Autodesk Inventor part; units mm, degrees
ref_plane "YZ Plane" through (0, 0, 0) normal (1, 0, 0) x (0, 1, 0)
ref_plane "XZ Plane" through (0, 0, 0) normal (0, 1, 0) x (-1, 0, 0)
ref_plane "XY Plane" through (0, 0, 0) normal (0, 0, 1) x (1, 0, 0)
sketch "Sketch1" plane through (0, 0, 0) normal (1, 0, 0) x (0, 1, 0)
  line L0 (0, 0) -> (185.293, 0)
  line L1 (0, 10.922) -> (185.293, 10.922)
  line L2 (0, 10.922) -> (0, 9.779) construction
  line L3 (0, 9.779) -> (185.293, 9.779)
  line L4 (185.293, 9.779) -> (185.293, 10.922) construction
  line L5 (0, 9.779) -> (0, 0) construction
  line L6 (185.293, 9.779) -> (185.293, 0) construction
  line L7 (0, 9.779) -> (1.143, 10.922)
  line L8 (185.293, 9.779) -> (184.15, 10.922)
  line L9 (0, 9.779) -> (0, 8.89)
  line L10 (0, 8.89) -> (3.175, 8.89)
  line L11 (3.175, 8.89) -> (3.175, 9.779)
  dimension "d0" = 185.293
  dimension "d2" = 19.558
  dimension "d3" = 45
  dimension "d5" = 21.844
  dimension "d6" = 3.175
  dimension "d7" = 17.78
revolve "Revolution1" add sketch "Sketch1" angle 360 about axis through (0, 0, 0) along (0, 1, 0)
properties part number "Rebuild Shooter NCDME075-0600 Body" material "Stainless Steel"
Check sheet for the modelled part. Datum: model origin and axes. Units: mm. Coordinates: 2 decimals unless noted, no trailing zeros. Order: outer loops, then holes, each group sorted by start corner. A loop starts at its lowest first (then second) coordinate and runs counter-clockwise, first axis right, second up. Notation, with made-up numbers: (18.5, -36.5) -> (70.5, -36.5) arc R34 ccw to (70.5, -2.5) -> close; hole circle Ø7 at (74.5, 61.5). An arc over 180 degrees is marked (long way). Write item = value, one per line. Start each with the question number.
1) Go/stop test with flat-tipped pins: P1, Ø4, axis at x = 8.5, z = 8.5, coming from the +Y side; P2, Ø2, axis at x = 6.5, y = 105.5, coming from the -Z side; P3, Ø3, axis at y = 146, z = 6.5, coming from the -X side. Record where each tip stops, or that it passes through.
2) Mould release check, pull along Z, two halves, no side actions. Record for faces 1 (the cylindrical face through (3.281, 93.928, 10.418)), 2 (the flat face through (-9, 0, 2)), 3 (the flat face through (-9, 3.175, 2)), 4 (the cylindrical face through (-8.68, 1.61, -1.93)): +Z half, -Z half, draft (parallel to the pull), parting line (faces both ways), or undercut.
3) Material ranges on L1, parallel to X at y = 26, z = -0.25; L2, parallel to Y at x = 9, z = 0 (3 decimals); L3, parallel to X at y = 108, z = -5, recorded low to high.
4) Cross-section at A-A (x = 0). Enter the section's corners in (y, z) (3 decimals), then the cut area to 3 significant figures.
5) Cross-section at B-B (z = 0). Enter the section's corners in (x, y) (3 decimals).
6) Cross-section at C-C (y = 98.5). Enter the section's corners in (x, z), then the cut area to 3 significant figures.
Ans:
q1.P1 = 185.05
q1.P2 = -9.44
q1.P3 = -9.71
q2.face_1 = parting line
q2.face_2 = draft
q2.face_3 = undercut
q2.face_4 = undercut
q3.L1 = -10.92 to -9.78, 9.78 to 10.92
q3.L2 = 0 to 3.175
q3.L3 = -9.71 to -8.4, 8.4 to 9.71
q4.outline = (0, -9.779) -> (1.143, -10.922) -> (184.15, -10.922) -> (185.293, -9.779) -> (3.175, -9.779) -> (3.175, -8.89) -> (0, -8.89) -> close; (0, 8.89) -> (3.175, 8.89) -> (3.175, 9.779) -> (185.293, 9.779) -> (184.15, 10.922) -> (1.143, 10.922) -> (0, 9.779) -> close
q4.area = 427 mm²
q5.outline = (-10.922, 1.143) -> (-9.779, 0) -> (-8.89, 0) -> (-8.89, 3.175) -> (-9.779, 3.175) -> (-9.779, 185.293) -> (-10.922, 184.15) -> close; (8.89, 0) -> (9.779, 0) -> (10.922, 1.143) -> (10.922, 184.15) -> (9.779, 185.293) -> (9.779, 3.175) -> (8.89, 3.175) -> close
q6.outline = circle Ø21.84 at (0, 0); hole circle Ø19.56 at (0, 0)
q6.area = 74.3 mm²
